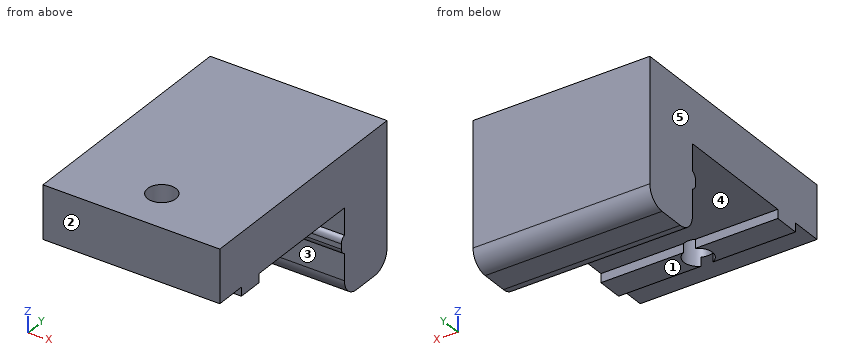
from build123d import *

# Parameters (mm, degrees)
ESQUISSE1_W             = 20
ESQUISSE1_H             = 27.5
BOSS_EXTRU_1_DEPTH      = 6
ESQUISSE2_W             = 20
ESQUISSE2_H             = 7
BOSS_EXTRU_2_DEPTH      = 10
CONG_2_R                = 2
ESQUISSE3_W             = 20
ESQUISSE3_H             = 2.9
BOSS_EXTRU_3_DEPTH      = 1
ESQUISSE4_R             = 1.6
ENL_V_MAT_EXTRU_1_DEPTH = 24.346573624
ESQUISSE6_W             = 20
ESQUISSE6_H             = 2
BOSS_EXTRU_5_DEPTH      = 0.5
CONG_4_R                = 0.75


with BuildPart() as part:
    # Esquisse1 → Boss.-Extru.1 (new body)
    with BuildSketch(Plane.XY):
        Rectangle(ESQUISSE1_W, ESQUISSE1_H)
    extrude(amount=BOSS_EXTRU_1_DEPTH)

    # Esquisse2 → Boss.-Extru.2 (add)
    with BuildSketch(Plane(origin=(0, 0, 0), x_dir=(-1, 0, 0), z_dir=(0, 0, -1))):
        with Locations((0, 10.25)):
            Rectangle(ESQUISSE2_W, ESQUISSE2_H)
    extrude(amount=BOSS_EXTRU_2_DEPTH)

    # Congé2
    cong_2_edges = [part.edges().sort_by_distance(p)[0] for p in [
        (0, 6.75, -10),
        (0, 13.75, -10),
    ]]
    fillet(cong_2_edges, radius=CONG_2_R)

    # Esquisse3 → Boss.-Extru.3 (add)
    with BuildSketch(Plane(origin=(0, 0, 0), x_dir=(-1, 0, 0), z_dir=(0, 0, -1))):
        with Locations((0, -8.75)):
            Rectangle(ESQUISSE3_W, ESQUISSE3_H)
    extrude(amount=BOSS_EXTRU_3_DEPTH)

    # Esquisse4 → Enlèv. mat.-Extru.1 (cut, through all)
    with BuildSketch(Plane.XY.offset(6)):
        with Locations((0, -8.75)):
            Circle(ESQUISSE4_R)
    extrude(amount=-ENL_V_MAT_EXTRU_1_DEPTH, mode=Mode.SUBTRACT)

    # Esquisse6 → Boss.-Extru.5 (add)
    with BuildSketch(Plane.XZ.offset(-6.75)):
        with Locations((0, -4)):
            Rectangle(ESQUISSE6_W, ESQUISSE6_H)
    extrude(amount=BOSS_EXTRU_5_DEPTH)

    # Congé4
    # the kernel refuses this fillet: 0.75 mm, written as the material it takes off along each edge
    with BuildSketch(Plane(origin=(-11.767766953, 6.25, -5), x_dir=(0, 1, 0), z_dir=(1, 0, 0)), Plane(origin=(11.767766953, 6.25, -3), x_dir=(0, 1, 0), z_dir=(-1, 0, 0))) as cong_4_piece_1:
        with BuildLine():
            CenterArc((0.75, 0.707106781), CONG_4_R, 180, 70.528779366)
            Line((0, 0.707106781), (-0.015, 0.707106781))
            Line((-0.015, 0.707106781), (-0.015, 0))
            Line((-0.015, 0), (0, -0.015))
            ThreePointArc((0, -0.015), (0.25, -0.015), (0.495, -0.014142136))
            Line((0.495, -0.014142136), (0.5, 0))
        make_face()
    extrude(amount=23.535533906, mode=Mode.SUBTRACT)


solid = part.part
Geometry: final body of the model. Coordinates: model frame, mm. Face numbers are marked on the shaded views. A direction names the side the tool comes from. Round coordinates to 2 decimals unless told otherwise and drop trailing zeros. Loops run counter-clockwise (first coordinate to the right, second up) from the corner with the lowest first, then second, coordinate; pieces in that order, holes last. Notation, with made-up numbers: (68.5, 58.5) -> (123.5, 58.5) arc R8 ccw to (123.5, 67.5) -> close; hole circle Ø3 at (68, 10). An arc over 180 degrees is marked (long way). One line per question, with ' | ' between items. Start each with the question number.
1. Contact query for flat-ended pins moving along their axis: pin 1 (1.1 mm diameter, centred on x = -5, z = -0.5, fed in from -Y); pin 2 (8 mm diameter, centred on x = 0, z = -5.5, fed in from -Y); pin 3 (4 mm diameter, centred on x = -4.5, y = -7, fed in from -Z); pin 4 (1 mm diameter, centred on x = -4, y = 2, fed in from -Z). Output: stop coordinate, or through.
2. Section B-B on x = 0. Output: boundary loops of the cut face in (y, z), and give its area (3 significant figures).
3. Section D-D on z = -1.75. Output: boundary loops of the cut face in (x, y).
4. Line query: line 1 along Y through (x, z) = (0, 1.5); line 2 along Z through (x, y) = (-0.75, -7); line 3 along X through (y, z) = (-10, 1). Output: solid intervals per line, ascending. Write a range as [from, to].
5. Section A-A on y = -8.75. Output: boundary loops of the cut face in (x, z).
6. Mould query, pull axis Y, two halves, no side actions, for the marked faces 3, 4 and 5. Classes: pulls with the +Y half, pulls with the -Y half, needs draft (parallel to the pull), parting line crosses it, or undercut.
7. Section C-C on x = 7. Output: boundary loops of the cut face in (y, z), and give its area (3 significant figures).
8. Set-up query: the marked faces 1 and 2. Return all of +Z, -Z, +X, -X, +Y, -Y with unobstructed straight access to the full face (end or side cutting, diameter ignored); none if empty.
Returned:
1) pin 1: stops at y = -13.75 | pin 2: stops at y = 6.25 | pin 3: stops at z = -1 | pin 4: stops at z = 0
2) outline: (-13.75, 0) -> (-10.35, 0) -> (-10.35, 6) -> (-13.75, 6) -> close; (-7.15, 0) -> (6.75, 0) -> (6.75, -3) arc R0.75 ccw to (6.25, -3.71) -> (6.25, -4.29) arc R0.75 ccw to (6.75, -5) -> (6.75, -8) arc R2 ccw to (8.75, -10) -> (11.75, -10) arc R2 ccw to (13.75, -8) -> (13.75, 6) -> (-7.15, 6) -> close | area: 215 mm2
3) outline: (-10, 6.75) -> (10, 6.75) -> (10, 13.75) -> (-10, 13.75) -> close
4) line 1: y = [-13.75, -10.35], [-7.15, 13.75] | line 2: z = [0, 6] | line 3: x = [-10, -1], [1, 10]
5) outline: (-10, -1) -> (-1.6, -1) -> (-1.6, 6) -> (-10, 6) -> close; (1.6, -1) -> (10, -1) -> (10, 6) -> (1.6, 6) -> close
6) face 3: pulls with the -Y half | face 4: undercut | face 5: needs draft
7) outline: (-13.75, 0) -> (-10.2, 0) -> (-10.2, -1) -> (-7.3, -1) -> (-7.3, 0) -> (6.75, 0) -> (6.75, -3) arc R0.75 ccw to (6.25, -3.71) -> (6.25, -4.29) arc R0.75 ccw to (6.75, -5) -> (6.75, -8) arc R2 ccw to (8.75, -10) -> (11.75, -10) arc R2 ccw to (13.75, -8) -> (13.75, 6) -> (-13.75, 6) -> close | area: 237 mm2
8) face 1: -Z, +X, -X, -Y | face 2: +Z, -Z, +X, -X, -Y
